CAD build for the part. Positions are in the model's coordinates, mm. Coordinates: 2 decimals unless noted, no trailing zeros. Write each loop counter-clockwise with the first axis right and the second up, starting at its lowest first coordinate (ties: lowest second). Pieces come first, ordered by that corner, then holes. Notation, with made-up numbers: (4.25, 48) - (9.25, 48) arc R9 cw to (9.25, 52) - close; hole circle Ø11 at (14.25, 63.5). An arc over 180 degrees is marked (long way). Answer in a Markdown table with one row per item. Add a question column.
Q1. Band-saw the part on C-C (x = 0.35). State how many separate pieces and enclosed holes the cut face has, and give its area (3 significant figures).
Q2. Band-saw the part on B-B (y = -103). List the corners of the cut face in (x, z).
Q3. Drill centre line: line 1 along Z through (x, y) = (0.35, 10). Where is it in solid material? Low to high. Write a range as from..to.
Q4. Band-saw the part on A-A (z = -67.5). List the corners of the cut face in (x, y).
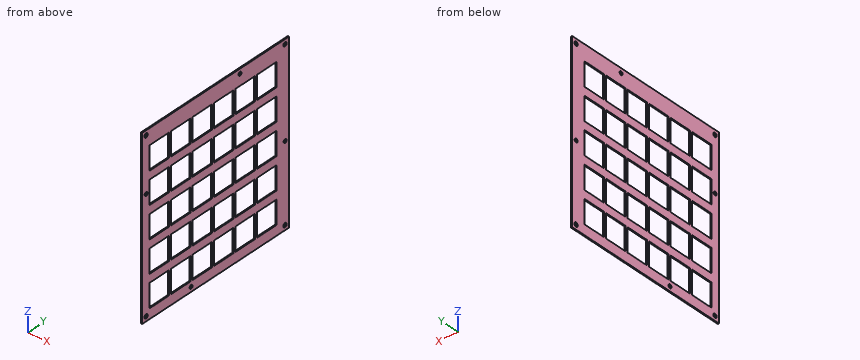
```python
from build123d import *

# Parameters (mm, degrees)
SKETCH2_W            = 150
SKETCH2_H            = 150
BOSS_EXTRUDE1_DEPTH  = 1
SKETCH4_W            = 20
SKETCH4_H            = 20
CUT_EXTRUDE1_DEPTH   = 160.418359102
LPATTERN1_COUNT      = 5
LPATTERN1_PITCH      = 27
LPATTERN1_COUNT_DIR2 = 6
LPATTERN1_PITCH_DIR2 = 22
M3_CLEARANCE_HOLE1_D = 3.4
SKETCH8_R            = 1.5
CUT_EXTRUDE2_DEPTH   = 160.418359102


with BuildPart() as part:
    # Sketch2 → Boss-Extrude1 (new body)
    with BuildSketch(Plane(origin=(0, 0, 0), x_dir=(0, 0, -1), z_dir=(1, 0, 0))):
        with Locations((34.101040119, -41.233283804)):
            Rectangle(SKETCH2_W, SKETCH2_H)
    extrude(amount=BOSS_EXTRUDE1_DEPTH)

    # Sketch4 → Cut-Extrude1 (cut, through all)
    with BuildSketch(Plane(origin=(1, 0, 0), x_dir=(0, 0, -1), z_dir=(1, 0, 0))):
        with Locations((-17.398959881, 11.266716196)):
            Rectangle(SKETCH4_W, SKETCH4_H)
    cut_extrude1 = extrude(amount=-CUT_EXTRUDE1_DEPTH, mode=Mode.SUBTRACT)

    # LPattern1: Cut-Extrude1 5 × 6
    with Locations(*[(0, -j * LPATTERN1_PITCH_DIR2, -i * LPATTERN1_PITCH) for i in range(LPATTERN1_COUNT) for j in range(LPATTERN1_COUNT_DIR2) if (i, j) != (0, 0)]):
        add(cut_extrude1, mode=Mode.SUBTRACT)

    # M3 Clearance Hole1 (through all)
    with Locations(Plane(origin=(1, 0, 0), x_dir=(0, 0, -1), z_dir=(1, 0, 0))):
        with Locations((-36.898959881, 29.766716196), (105.101040119, 29.766716196), (105.101040119, -112.233283804), (-36.898959881, -112.233283804)):
            Hole(M3_CLEARANCE_HOLE1_D / 2)

    # Sketch8 → Cut-Extrude2 (cut, through all)
    with BuildSketch(Plane(origin=(1, 0, 0), x_dir=(0, 0, -1), z_dir=(1, 0, 0))):
        with Locations((39.101040119, 29.766716196)):
            Circle(SKETCH8_R)
        with Locations((-36.898959881, -16.233283804)):
            Circle(SKETCH8_R)
        with Locations((9.101040119, -112.233283804)):
            Circle(SKETCH8_R)
        with Locations((105.101040119, -66.233283804)):
            Circle(SKETCH8_R)
    extrude(amount=-CUT_EXTRUDE2_DEPTH, mode=Mode.SUBTRACT)


solid = part.part
```
Checked values:
| question | item | result |
|---|---|---|
| 1 | separate pieces | 1 |
| 1 | enclosed holes | 38 |
| 1 | area | 10,400 mm² |
| 2 | outline | (0, -109.1) - (1, -109.1) - (1, -100.6) - (0, -100.6) - close; (0, -80.6) - (1, -80.6) - (1, -73.6) - (0, -73.6) - close; (0, -53.6) - (1, -53.6) - (1, -46.6) - (0, -46.6) - close; (0, -26.6) - (1, -26.6) - (1, -19.6) - (0, -19.6) - close; (0, 0.4) - (1, 0.4) - (1, 7.4) - (0, 7.4) - close; (0, 27.4) - (1, 27.4) - (1, 40.9) - (0, 40.9) - close |
| 3 | line 1 | z = -109.1..-100.6, -80.6..-73.6, -53.6..-46.6, -26.6..-19.6, 0.4..7.4, 27.4..40.9 |
| 4 | outline | (0, -116.23) - (1, -116.23) - (1, -108.73) - (0, -108.73) - close; (0, -88.73) - (1, -88.73) - (1, -86.73) - (0, -86.73) - close; (0, -66.73) - (1, -66.73) - (1, -64.73) - (0, -64.73) - close; (0, -44.73) - (1, -44.73) - (1, -42.73) - (0, -42.73) - close; (0, -22.73) - (1, -22.73) - (1, -20.73) - (0, -20.73) - close; (0, -0.73) - (1, -0.73) - (1, 1.27) - (0, 1.27) - close; (0, 21.27) - (1, 21.27) - (1, 33.77) - (0, 33.77) - close |
